The model under review builds one solid part; all positions refer to its coordinate system, in mm. A direction names the side the tool comes from. Give positions to 0.01 mm unless a question says otherwise; leave off trailing zeros. Order: outer loops, then holes, each group sorted by start corner. A loop starts at its lowest first (then second) coordinate and runs counter-clockwise, first axis right, second up.
```python
from build123d import *

# Parameters (mm, degrees)
PAD008_DEPTH    = 4
SKETCH032_R     = 3.05
POCKET_DEPTH    = 3.2
SKETCH033_R     = 5
POCKET001_DEPTH = 1


with BuildPart() as part:
    # Sketch013 → Pad008 (new body)
    with BuildSketch(Plane(origin=(0, 0, 0), x_dir=(-1, 0, 0), z_dir=(0, 1, 0))):
        with BuildLine():
            Line((-6, 11), (6, 11))
            ThreePointArc((11, 6), (9.535534, 9.535534), (6, 11))
            Line((11, 6), (11, -6))
            ThreePointArc((6, -11), (9.535534, -9.535534), (11, -6))
            Line((6, -11), (-6, -11))
            ThreePointArc((-11, -6), (-9.535534, -9.535534), (-6, -11))
            Line((-11, -6), (-11, 6))
            ThreePointArc((-6, 11), (-9.535534, 9.535534), (-11, 6))
        make_face()
    extrude(amount=PAD008_DEPTH)

    # Sketch032 → Pocket (cut)
    with BuildSketch(Plane.XZ):
        Circle(SKETCH032_R)
    extrude(amount=-POCKET_DEPTH, mode=Mode.SUBTRACT)

    # Sketch033 (on Face5 of Pocket) → Pocket001 (cut)
    with BuildSketch(Plane(origin=(0, 4, 0), x_dir=(1, 0, 0), z_dir=(0, 1, 0))):
        Circle(SKETCH033_R)
    extrude(amount=-POCKET001_DEPTH, mode=Mode.SUBTRACT)


with BuildPart() as part_1:
    # Body013 placement: moved
    add(part.part.moved(Location((0, 110, 0))))


solid = part_1.part
```
Item 1: Take a section at C-C (z = 0). Give the boundary of the cut face in (x, y).
Values found:
outline: (-11, 110) - (-3.05, 110) - (-3.05, 113) - (-5, 113) - (-5, 114) - (-11, 114) - close; (3.05, 110) - (11, 110) - (11, 114) - (5, 114) - (5, 113) - (3.05, 113) - close
Item 2: Take a section at A-A (x = 0). Give the boundary of the cut face in (y, z).
Values found:
outline: (110, -11) - (114, -11) - (114, -5) - (113, -5) - (113, -3.05) - (110, -3.05) - close; (110, 3.05) - (113, 3.05) - (113, 5) - (114, 5) - (114, 11) - (110, 11) - close
Item 3: For line 1 (Z direction, x = 0, y = 113.65); line 2 (Z direction, x = 0, y = 110.8); line 3 (X direction, y = 112.65, z = -1.75), list the stretches that pass through material, from the lowest coordinate up.
Values found:
line 1: z = -11 to -5, 5 to 11
line 2: z = -11 to -3.05, 3.05 to 11
line 3: x = -11 to -2.5, 2.5 to 11
Item 4: Take a section at B-B (y = 112.5). Give the boundary of the cut face in (x, z), and give its area (3 significant figures).
Values found:
outline: (-11, -6) arc R5 ccw to (-6, -11) - (6, -11) arc R5 ccw to (11, -6) - (11, 6) arc R5 ccw to (6, 11) - (-6, 11) arc R5 ccw to (-11, 6) - close; hole circle Ø6.1 at (0, 0)
area: 433 mm2
Item 5: For faces 1 (the cylindrical face through (-1.08, 113.51, 4.88)), 2 (the cylindrical face through (-9, 112, -10)), list the 3-axis set-ups (+Z, -Z, +X, -X, +Y, -Y) from which the entire face can be reached by the end or side of a thin tool; tool diameter is ignored.
Values found:
face 1: +Y
face 2: -Z, -X, +Y, -Y
Item 6: Draft analysis for pull direction X (two halves, no side actions). For faces 3 (the cylindrical face through (-10, 112, 9)), 4 (the flat face through (-0.1, 113, 3.3)), 5 (the cylindrical face through (10, 112, -9)), 6 (the flat face through (-3, 114, 5)), state which applies: released by +X, released by -X, zero draft, split by the parting line, or undercut.
Values found:
face 3: released by -X
face 4: undercut
face 5: released by +X
face 6: zero draft
Item 7: Clearance check with a flat-ended pin moving along its axis: pin 1 Ø3 at (x, z) = (-2, 1.5) entering from +Y. State where the tip first meets the part, or that it passes through.
Values found:
pin 1: stops at y = 113
Item 8: Take a section at D-D (z = -4.5). Give the boundary of the cut face in (x, y), and give its area (3 significant figures).
Values found:
outline: (-11, 110) - (11, 110) - (11, 114) - (2.18, 114) - (2.18, 113) - (-2.18, 113) - (-2.18, 114) - (-11, 114) - close
area: 83.6 mm2
